Work out the finished part from the listing and answer in its coordinate system (mm). A direction names the side the tool comes from. Give positions to 0.01 mm unless a question says otherwise; leave off trailing zeros. Order: outer loops, then holes, each group sorted by start corner. A loop starts at its lowest first (then second) coordinate and runs counter-clockwise, first axis right, second up.
```python
from build123d import *

# Parameters (mm, degrees)
SKETCH1_W           = 17
SKETCH1_H           = 15
BOSS_EXTRUDE1_DEPTH = 1
CHAMFER1_SIZE       = 2.5
BOSS_EXTRUDE2_START = 1
SKETCH2_W           = 5
SKETCH2_H           = 3.5
BOSS_EXTRUDE2_DEPTH = 1
SKETCH3_R           = 1
SKETCH3_R_2         = 0.5
CUT_EXTRUDE1_DEPTH  = 1
SKETCH4_W           = 2
SKETCH4_H           = 1.2
SKETCH4_W_2         = 0.5
SKETCH4_W_3         = 1.5
SKETCH4_H_2         = 0.8
BOSS_EXTRUDE3_DEPTH = 0.5
SKETCH5_W           = 3
SKETCH5_H           = 1.5
CUT_EXTRUDE2_DEPTH  = 0.01


with BuildPart() as part:
    # Sketch1 → Boss-Extrude1 (new body)
    with BuildSketch(Plane.XY):
        Rectangle(SKETCH1_W, SKETCH1_H)
    extrude(amount=BOSS_EXTRUDE1_DEPTH)

    # Chamfer1
    chamfer1_edges = [part.edges().sort_by_distance(p)[0] for p in [
        (8.5, -7.5, 0.5),
        (-8.5, -7.5, 0.5),
        (-8.5, 7.5, 0.5),
        (8.5, 7.5, 0.5),
    ]]
    chamfer(chamfer1_edges, length=CHAMFER1_SIZE)

    # Sketch2 → Boss-Extrude2 (add)
    with BuildSketch(Plane.XY.offset(BOSS_EXTRUDE2_START)):
        Rectangle(SKETCH2_W, SKETCH2_H)
    extrude(amount=BOSS_EXTRUDE2_DEPTH)

    # Sketch3 → Cut-Extrude1 (cut)
    with BuildSketch(Plane.XY):
        with Locations((0, 5.5)):
            Circle(SKETCH3_R)
        with Locations((0, -5.5)):
            Circle(SKETCH3_R)
        with Locations((6.5, 0)):
            Circle(SKETCH3_R_2)
        with Locations((-6.5, 0)):
            Circle(SKETCH3_R_2)
        with Locations((6.5, 2)):
            Circle(SKETCH3_R_2)
        with Locations((6.5, 4)):
            Circle(SKETCH3_R_2)
        with Locations((-6.5, 2)):
            Circle(SKETCH3_R_2)
        with Locations((-6.5, -2)):
            Circle(SKETCH3_R_2)
        with Locations((6.5, -4)):
            Circle(SKETCH3_R_2)
        with Locations((6.5, -2)):
            Circle(SKETCH3_R_2)
    extrude(amount=CUT_EXTRUDE1_DEPTH, mode=Mode.SUBTRACT)

    # Sketch4 → Boss-Extrude3 (add)
    with BuildSketch(Plane.XY):
        with Locations((-0.618205111, -2.566679178)):
            Rectangle(SKETCH4_W, SKETCH4_H)
        with Locations((-2.420773885, -4.883367435)):
            Rectangle(SKETCH4_W_2, SKETCH4_H)
        with Locations((3.286986257, -4.838471609)):
            Rectangle(SKETCH4_W_3, SKETCH4_H_2)
    extrude(amount=-BOSS_EXTRUDE3_DEPTH)

    # Sketch5 → Cut-Extrude2 (cut)
    with BuildSketch(Plane.XY):
        with Locations((6.5, -4)):
            Rectangle(SKETCH5_W, SKETCH5_H)
        with Locations((6.5, -2)):
            Rectangle(SKETCH5_W, SKETCH5_H)
        with Locations((6.5, 0)):
            Rectangle(SKETCH5_W, SKETCH5_H)
        with Locations((6.5, 2)):
            Rectangle(SKETCH5_W, SKETCH5_H)
        with Locations((6.5, 4)):
            Rectangle(SKETCH5_W, SKETCH5_H)
        with Locations((-6.5, -2)):
            Rectangle(SKETCH5_W, SKETCH5_H)
        with Locations((-6.5, 0)):
            Rectangle(SKETCH5_W, SKETCH5_H)
        with Locations((-6.5, 2)):
            Rectangle(SKETCH5_W, SKETCH5_H)
    extrude(amount=CUT_EXTRUDE2_DEPTH, mode=Mode.SUBTRACT)


solid = part.part
```
1. The part is cut by section C-C (y = 0). State how many separate pieces and enclosed holes the cut face has, then the cut area to 3 significant figures.
Findings below:
separate pieces: 3
enclosed holes: 0
area: 20.0 mm2
2. Straight lines are drawn through the part: probe 1 along Y at (x, z) = (6.5, 0.65); probe 2 along X at (y, z) = (-2, 0.8); probe 3 along Z at (x, y) = (5.5, -2). For each, find the intervals that lie inside material, in ascending order.
Findings below:
probe 1: y = -7 to -4.5, -3.5 to -2.5, -1.5 to -0.5, 0.5 to 1.5, 2.5 to 3.5, 4.5 to 7
probe 2: x = -8.5 to -7, -6 to 6, 7 to 8.5
probe 3: z = 0.01 to 1
3. The mould has two halves that part along X. Classify faces 3 (the face through (-2.5, 0, 1.5)), 4 (the face through (0, -1.75, 1.5)), 5 (the face through (-0.13, -4.51, 0.49)): pulls with the +X half, pulls with the -X half, needs draft (parallel to the pull), parting line crosses it, or undercut.
Findings below:
face 3: pulls with the -X half
face 4: needs draft
face 5: undercut
4. The part is cut by section B-B (x = 0). Write down the section's boundary in (y, z).
Findings below:
outline: (-7.5, 0) - (-6.5, 0) - (-6.5, 1) - (-7.5, 1) - close; (-4.5, 0) - (-3.17, 0) - (-3.17, -0.5) - (-1.97, -0.5) - (-1.97, 0) - (4.5, 0) - (4.5, 1) - (1.75, 1) - (1.75, 2) - (-1.75, 2) - (-1.75, 1) - (-4.5, 1) - close; (6.5, 0) - (7.5, 0) - (7.5, 1) - (6.5, 1) - close
5. Given P1, Ø1.2, axis at x = -6, y = 0, coming from the -Z side; P2, Ø2.5, axis at x = 0, y = -5.5, coming from the +Z side, each flat-ended and moving along its own axis, determine where each tip first touches the part or whether it passes through.
Findings below:
P1: stops at z = 0.01
P2: stops at z = 1
6. Which of the six approach directions +Z, -Z, +X, -X, +Y, -Y give full straight-line access (tool end or side, diameter ignored) to faces 1 (the face through (0, 1.75, 1.5)), 2 (the face through (-1, -3, -0.5))?
Findings below:
face 1: +Z, +X, -X, +Y
face 2: -Z, +X, -X, +Y, -Y
